For this review, take the finished solid that the model builds, in its own axes (mm). A direction names the side the tool comes from. Give positions to 0.01 mm unless a question says otherwise; leave off trailing zeros. Write each loop counter-clockwise with the first axis right and the second up, starting at its lowest first coordinate (ties: lowest second). Pieces come first, ordered by that corner, then holes. Notation, with made-up numbers: (-28.75, 51) -> (26.25, 51) arc R14 ccw to (26.25, 65) -> close; hole circle Ø4 at (-27, 22.5). An arc over 180 degrees is marked (long way). Write item = value, one per line.
```python
from build123d import *

# Parameters (mm, degrees)
F1_DEPTH  = 12.7
F2_SIZE   = 19.05
F3_R      = 7.9375
F3_R_2    = 6.35
F4_DEPTH  = 74.422
F3_W      = 12.7
F3_H      = 120.65
F5_DEPTH  = 107.95
F6_SIZE   = 19.05
F7_R      = 19.05
F8_DEPTH  = 399.034
F3_W_2    = 72.2113
F3_H_2    = 9.525
F9_DEPTH  = 76.2
F11_DEPTH = 180.848


with BuildPart() as f1:
    # F0 (on Front) → F1 (new body)
    with BuildSketch(Plane.XZ):
        Polygon((109.076549, 47.385406), (-58.384751, 47.385406), (-113.173451, -35.164594), (-113.173451, -73.264594), (109.076549, -73.264594), align=None)
    extrude(amount=F1_DEPTH)

    # F2
    f2_edges = [f1.edges().sort_by_distance(p)[0] for p in [
        (109.076549, -6.35, -73.264594),
        (109.076549, -6.35, 47.385406),
    ]]
    chamfer(f2_edges, length=F2_SIZE)

    # F3 (on face) → F4 (cut)
    with BuildSketch(Plane.XZ.offset(12.7)):
        with Locations((-10.759751, 21.985406)):
            Circle(F3_R)
        with Locations((78.140249, 21.985406)):
            Circle(F3_R_2)
        with Locations((78.140249, -54.214594)):
            Circle(F3_R_2)
        with Locations((-106.009751, -57.58049)):
            Circle(F3_R_2)
        with Locations((-10.759751, -54.214594)):
            Circle(F3_R)
    extrude(amount=-F4_DEPTH, mode=Mode.SUBTRACT)

    # F3 (on face) → F5 (join)
    with BuildSketch(Plane.XZ.offset(12.7)):
        with Locations((-52.034751, -12.939594)):
            Rectangle(F3_W, F3_H)
        Polygon((36.865249, 47.385406), (24.165249, 47.385406), (24.165249, -73.264594), (36.865249, -73.264594), (36.865249, -25.639594), (36.865249, -16.114594), align=None)
    extrude(amount=F5_DEPTH)

    # F6
    f6_edges = [f1.edges().sort_by_distance(p)[0] for p in [
        (30.515249, -120.65, 47.385406),
        (-52.034751, -120.65, 47.385406),
    ]]
    chamfer(f6_edges, length=F6_SIZE)

    # F7 (on face) → F8 (cut)
    with BuildSketch(Plane.YZ.offset(36.865249)):
        with Locations((-82.55, 9.285406)):
            Circle(F7_R)
        Polygon((-38.1, -73.264594), (-120.65, -9.764594), (-120.65, -73.264594), align=None)
    extrude(amount=-F8_DEPTH, mode=Mode.SUBTRACT)

    # F3 (on face) → F9 (join)
    with BuildSketch(Plane.XZ.offset(12.7)):
        with Locations((72.970899, -20.877094)):
            Rectangle(F3_W_2, F3_H_2)
    extrude(amount=F9_DEPTH)

    # F10 (on face) → F11 (cut)
    with BuildSketch(Plane(origin=(0, 0, -25.639594), x_dir=(1, 0, 0), z_dir=(0, 0, -1))):
        Polygon((109.076549, 88.9), (49.565249, 88.9), (109.076549, 25.4), align=None)
    extrude(amount=-F11_DEPTH, mode=Mode.SUBTRACT)


solid = f1.part
```
(1) For pin 1 (10.5 mm diameter, centred on x = 42.5, z = -20.5, fed in from -Y); pin 2 (12 mm diameter, centred on x = 77, y = -45.5, fed in from +Z); pin 3 (4 mm diameter, centred on x = -9, y = -15, fed in from +Z); pin 4 (3 mm diameter, centred on y = -68.5, z = -35, fed in from -X), all flat-tipped, find the tip position at first contact; note any pin that passes through.
Answers below:
pin_1 = -88.9
pin_2 = -16.11
pin_3 = through
pin_4 = -58.38
(2) Take a section at B-B (y = -86). Write out the cut boundary in (x, z), plus the area to 3 significant figures.
Answers below:
outline = (-58.38, -36.42) -> (-45.68, -36.42) -> (-45.68, -9.45) -> (-58.38, -9.45) -> close; (-58.38, 28.02) -> (-45.68, 28.02) -> (-45.68, 47.39) -> (-58.38, 47.39) -> close; (24.17, -36.42) -> (36.87, -36.42) -> (36.87, -25.64) -> (52.28, -25.64) -> (52.28, -16.11) -> (36.87, -16.11) -> (36.87, -9.45) -> (24.17, -9.45) -> close; (24.17, 28.02) -> (36.87, 28.02) -> (36.87, 47.39) -> (24.17, 47.39) -> close
area = 1,320 mm^2
(3) Tool access review of faces 4 (the face through (-11, -12.7, -12)), 5 (the face through (-58.385, -54, 0)), 6 (the face through (72, -12.7, 16)), 7 (the face through (64, -42, -25.64)): name each direction out of +Z, -Z, +X, -X, +Y, -Y from which nothing blocks a thin tool from reaching the whole face with its end or side.
Answers below:
face_4 = +Z, -Z, -Y
face_5 = +Z, -Z, -X, -Y
face_6 = +Z, +X, -Y
face_7 = -Z, +X, -Y
(4) To check wall thickness, follow probe 1 along X at (y, z) = (-44, -43.5); probe 2 along X at (y, z) = (-6.5, 21); probe 3 along Y at (x, z) = (-66.5, -41). State the ranges of each line that lie inside material, in increasing order.
Answers below:
probe_1 = -58.38 to -45.68, 24.17 to 36.87
probe_2 = -75.9 to -18.64, -2.88 to 71.87, 84.41 to 109.08
probe_3 = -12.7 to 0
(5) Take a section at A-A (y = -17.5). Write out the cut boundary in (x, z).
Answers below:
outline = (-58.38, -73.26) -> (-45.68, -73.26) -> (-45.68, 47.39) -> (-58.38, 47.39) -> close; (24.17, -73.26) -> (36.87, -73.26) -> (36.87, -25.64) -> (109.08, -25.64) -> (109.08, -16.11) -> (36.87, -16.11) -> (36.87, 47.39) -> (24.17, 47.39) -> close
(6) Take a section at D-D (z = 40). Write out the cut boundary in (x, y), plus the area to 3 significant figures.
Answers below:
outline = (-63.29, -12.7) -> (-58.38, -12.7) -> (-58.38, -108.99) -> (-45.68, -108.99) -> (-45.68, -12.7) -> (24.17, -12.7) -> (24.17, -108.99) -> (36.87, -108.99) -> (36.87, -12.7) -> (97.41, -12.7) -> (97.41, 0) -> (-63.29, 0) -> close
area = 4,490 mm^2
(7) Take a section at C-C (x = 69). Write out the cut boundary in (y, z), plus the area to 3 significant figures.
Answers below:
outline = (-68.16, -25.64) -> (-12.7, -25.64) -> (-12.7, -73.26) -> (0, -73.26) -> (0, 47.39) -> (-12.7, 47.39) -> (-12.7, -16.11) -> (-68.16, -16.11) -> close
area = 2,060 mm^2
(8) The part is to be moulded in two halves that separate along X. For faces 1 (the face through (-52.124, -111.258, 37.727)), 2 (the face through (-100.144, -6.439, -60.013)), 3 (the face through (78.9, -57.6, -20.9)), say which applies: released by +X, released by -X, zero draft, split by the parting line, or undercut.
Answers below:
face_1 = zero draft
face_2 = undercut
face_3 = released by +X
